Design review of the part built by this model. Coordinates are the model's own, in mm. Round coordinates to 2 decimals unless told otherwise and drop trailing zeros. Order: outer loops, then holes, each group sorted by start corner. A loop starts at its lowest first (then second) coordinate and runs counter-clockwise, first axis right, second up. Notation, with made-up numbers: M -4.5,51.5 L 38.5,51.5 A17 ccw 38.5,68.5 Z; hole C 50.5,80 d11. An arc over 180 degrees is marked long. Use a Markdown table: item, result. Add a question column.
(1) For pin 1 (2 mm diameter, centred on x = -28.5, z = 0.5, fed in from +Y); pin 2 (4.5 mm diameter, centred on x = -42.29, y = 29.94, fed in from +Z); pin 3 (1.5 mm diameter, centred on x = -29.5, z = 3, fed in from -Y), all flat-tipped, find the tip position at first contact; note any pin that passes through.
(2) Take a section at A-A (z = 2.45). Write out the cut boundary in (x, y), then the cut area to 3 significant figures.
(3) Take a section at B-B (y = 62). Write out the cut boundary in (x, z), then the cut area to 3 significant figures.
(4) The part is to be moulded in two halves that separate along Y. For faces 1 (the face through (-43, 20, 4)), 2 (the face through (-40.901, 4.364, 2.028)), 3 (the face through (-48.796, 79.514, 1.972)), say which applies: released by +Y, released by -Y, zero draft, split by the parting line, or undercut.
(5) Take a section at C-C (x = -54). Write out the cut boundary in (y, z).
(6) To check wall thickness, follow probe 1 along Y at (x, z) = (-42, 2.7); probe 2 along Y at (x, z) = (-44.5, 1.4); probe 3 along Y at (x, z) = (-44, 1.5). State the ranges of each line that lie inside material, in increasing order. Write a range as from..to.
```python
from build123d import *

# Parameters (mm, degrees)
SKETCH1_R           = 50
BOSS_EXTRUDE1_DEPTH = 4
SKETCH4_R           = 2.5
CUT_EXTRUDE1_DEPTH  = 5
SKETCH5_R           = 1.5
CUT_EXTRUDE2_DEPTH  = 4


with BuildPart() as part:
    # Sketch1 → Boss-Extrude1 (new body)
    with BuildSketch(Plane.XY):
        with Locations((-42.286719292, 29.938997259)):
            Circle(SKETCH1_R)
    extrude(amount=BOSS_EXTRUDE1_DEPTH)

    # Sketch4 → Cut-Extrude1 (cut)
    with BuildSketch(Plane.XY.offset(4)):
        with Locations((-42.286719292, 29.938997259)):
            Circle(SKETCH4_R)
    extrude(amount=-CUT_EXTRUDE1_DEPTH, mode=Mode.SUBTRACT)

    # Sketch5 → Cut-Extrude2 (cut)
    with BuildSketch(Plane.XY.offset(4)):
        with Locations((-67.286719292, 29.938997259)):
            Circle(SKETCH5_R)
        with Locations((-42.286719292, 54.938997259)):
            Circle(SKETCH5_R)
        with Locations((-17.286719292, 29.938997259)):
            Circle(SKETCH5_R)
        with Locations((-42.286719292, 4.938997259)):
            Circle(SKETCH5_R)
    extrude(amount=-CUT_EXTRUDE2_DEPTH, mode=Mode.SUBTRACT)


solid = part.part
```
Verdict:
| question | item | result |
|---|---|---|
| 1 | pin 1 | stops at y = 78.28 |
| 1 | pin 2 | passes through |
| 1 | pin 3 | stops at y = -18.59 |
| 2 | outline | C -42.29,29.94 d100; hole C -67.29,29.94 d3; hole C -42.29,29.94 d5; hole C -42.29,4.94 d3; hole C -42.29,54.94 d3; hole C -17.29,29.94 d3 |
| 2 | area | 7,810 mm^2 |
| 3 | outline | M -80.65,0 L -3.92,0 L -3.92,4 L -80.65,4 Z |
| 3 | area | 307 mm^2 |
| 4 | face 1 | zero draft |
| 4 | face 2 | undercut |
| 4 | face 3 | split by the parting line |
| 5 | outline | M -18.67,0 L 78.55,0 L 78.55,4 L -18.67,4 Z |
| 6 | probe 1 | y = -20.06..3.47, 6.41..27.46, 32.42..53.47, 56.41..79.94 |
| 6 | probe 2 | y = -20.01..28.78, 31.1..79.89 |
| 6 | probe 3 | y = -20.03..28.12, 31.76..79.91 |
